Autodesk Inventor part; units mm, degrees
ref_plane "YZ Plane" through (0, 0, 0) normal (1, 0, 0) x (0, 1, 0)
ref_plane "XZ Plane" through (0, 0, 0) normal (0, 1, 0) x (-1, 0, 0)
ref_plane "XY Plane" through (0, 0, 0) normal (0, 0, 1) x (1, 0, 0)
sketch "Sketch1" plane through (0, 0, 0) normal (0, 1, 0) x (-1, 0, 0)
  line L0 (-23.8125, -82.566) -> (23.8125, -82.566)
  line L1 (23.8125, -82.566) -> (23.8125, 82.566)
  line L2 (23.8125, 82.566) -> (-23.8125, 82.566)
  line L3 (-23.8125, 82.566) -> (-23.8125, -82.566)
  line L4 (-23.8125, -82.566) -> (23.8125, 82.566) construction
  line L5 (23.8125, -82.566) -> (-23.8125, 82.566) construction
  point P0 (0, 0)
  dimension "d0" = 47.625
  dimension "d1" = 165.132
extrude "Extrusion1" add sketch "Sketch1" along normal blind 20.6248
sketch "Sketch5" plane through (-23.8125, 0, -82.566) normal (-1, 0, 0) x (0, 0, 1)
  line L0 (0, 20.6248) -> (165.132, 20.6248)
  line L1 (165.132, 0) -> (0, 0)
  line L2 (0, 20.6248) -> (165.132, 20.6248)
  line L3 (165.132, 20.6248) -> (165.132, 0)
  line L4 (165.132, 0) -> (0, 0)
  line L5 (0, 0) -> (0, 20.6248)
  point P0 (82.566, 0)
extrude "Extrusion4" add sketch "Sketch5" along normal blind 2.3495
sketch "Sketch6" plane through (23.8125, 0, 82.566) normal (1, 0, 0) x (0, 0, -1)
  line L0 (0, 0) -> (0, 20.6248)
  line L1 (0, 0) -> (165.132, 0)
  line L2 (0, 20.6248) -> (165.132, 20.6248)
  line L3 (165.132, 20.6248) -> (165.132, 0)
  line L4 (165.132, 0) -> (0, 0)
  line L5 (0, 0) -> (0, 20.6248)
  point P0 (82.566, 0)
extrude "Extrusion5" add sketch "Sketch6" along normal blind 2.3495
sketch "Sketch7" plane through (-26.162, 0, -82.566) normal (0, 0, -1) x (-1, 0, 0)
  line L0 (0, 0) -> (-52.324, 0)
  line L1 (0, -3.175) -> (3.175, -3.175)
  line L2 (0, -3.175) -> (0, 0)
  arc A0 (3.175, -3.175) -> (0, 0) centre (0, -3.175) ccw
  line L3 (-52.324, 0) -> (-52.324, -3.175)
  arc A1 (-52.324, 0) -> (-55.499, -3.175) centre (-52.324, -3.175) ccw
  line L4 (-52.324, -3.175) -> (-55.499, -3.175)
  line L5 (-52.324, 0) -> (-52.324, 6.35)
  line L6 (-52.324, 0) -> (-52.324, 20.6248)
  arc A2 (-52.324, 6.35) -> (-61.849, -3.175) centre (-52.324, -3.175) ccw
  line L7 (-55.499, -3.175) -> (-61.849, -3.175)
  line L8 (-55.499, -3.175) -> (-55.499, -10.795)
  line L9 (-55.499, -10.795) -> (-61.849, -10.795)
  line L10 (-61.849, -10.795) -> (-61.849, -3.175)
  line L11 (-55.499, -10.795) -> (-58.674, -10.795)
  arc A3 (-58.674, -13.97) -> (-55.499, -10.795) centre (-58.674, -10.795) ccw
  line L12 (-58.674, -13.97) -> (-66.294, -13.97)
  line L13 (-66.294, -13.97) -> (-66.294, -17.145)
  arc A4 (-66.294, -13.97) -> (-69.469, -17.145) centre (-66.294, -17.145) ccw
  line L14 (-66.294, -17.145) -> (-69.469, -17.145)
  line L15 (-69.469, -17.145) -> (-69.469, -22.225)
  line L16 (-61.849, -13.97) -> (-61.849, -7.62)
  line L17 (-61.849, -7.62) -> (-66.294, -7.62)
  arc A5 (-66.294, -7.62) -> (-75.819, -17.145) centre (-66.294, -17.145) ccw
  line L18 (-69.469, -22.225) -> (-75.819, -22.225)
  line L19 (-75.819, -22.225) -> (-75.819, -17.145)
  line L20 (-69.469, -17.145) -> (-75.819, -17.145)
  line L21 (-26.162, 0) -> (-26.162, 12.6356)
  arc A6 (3.175, -3.175) -> (0, 0) centre (0, -3.175) ccw
  line L22 (0, -3.175) -> (3.175, -3.175)
  arc A7 (9.525, -3.175) -> (0, 6.35) centre (0, -3.175) ccw
  line L23 (3.175, -3.175) -> (9.525, -3.175)
  line L24 (3.175, -3.175) -> (3.175, -10.795)
  line L25 (3.175, -10.795) -> (9.525, -10.795)
  line L26 (9.525, -10.795) -> (9.525, -3.175)
  line L27 (3.175, -10.795) -> (6.35, -10.795)
  arc A8 (3.175, -10.795) -> (6.35, -13.97) centre (6.35, -10.795) ccw
  line L28 (6.35, -13.97) -> (13.97, -13.97)
  line L29 (13.97, -13.97) -> (13.97, -17.145)
  arc A9 (17.145, -17.145) -> (13.97, -13.97) centre (13.97, -17.145) ccw
  line L30 (13.97, -17.145) -> (17.145, -17.145)
  line L31 (17.145, -17.145) -> (17.145, -22.225)
  line L32 (9.525, -13.97) -> (9.525, -7.62)
  line L33 (9.525, -7.62) -> (13.97, -7.62)
  arc A10 (23.495, -17.145) -> (13.97, -7.62) centre (13.97, -17.145) ccw
  line L34 (17.145, -22.225) -> (23.495, -22.225)
  line L35 (23.495, -22.225) -> (23.495, -17.145)
  line L36 (17.145, -17.145) -> (23.495, -17.145)
  line L37 (0, 20.6248) -> (0, 0)
  line L38 (0, 0) -> (0, 6.35)
  dimension "d22" = 3.175
  dimension "d23" = 6.35
  dimension "d24" = 7.62
  dimension "d26" = 7.62
  dimension "d29" = 3.175
  dimension "d30" = 5.08
  dimension "d31" = 6.35
  dimension "d32" = 6.35
extrude "Extrusion6" add sketch "Sketch7" against normal blind 158.75 contours A1 L7 A2 L5 | L37 A7 L23 A0 | L23 L26 L25 L24 | L25 L32 L28 A8 | L8 L9 L10 L7 | L33 A10 L36 A9 L28 L32 L26 | A3 L12 L16 L9 | L10 L16 L12 A4 L20 A5 L17 | L35 L34 L31 L36 | L20 L15 L18 L19
sketch "Sketch10" plane through (-26.162, 0, 82.566) normal (0, 0, 1) x (1, 0, 0)
  line L0 (26.162, 20.0804) -> (26.162, 7.3804)
  line L1 (26.162, 7.3804) -> (38.862, 7.3804)
  line L2 (26.162, 7.3804) -> (13.462, 7.3804)
  circle A0 centre (13.462, 7.3804) radius 3.5687
  circle A1 centre (38.862, 7.3804) radius 3.5687
  point P0 (26.162, 0)
  dimension "d52" = 12.7
  dimension "d53" = 12.7
  dimension "d54" = 12.7
  dimension "d55" = 7.1374
  dimension "d56" = 7.1374
extrude "Extrusion9" cut sketch "Sketch10" against normal blind 6.35
sketch "Sketch11" plane through (26.162, 20.6248, -82.566) normal (0, 0, -1) x (-1, 0, 0)
  line L0 (0, 0) -> (52.324, 0)
  line L1 (26.162, 0) -> (26.162, -12.7)
  line L2 (26.162, -12.7) -> (38.862, -12.7)
  line L3 (38.862, -12.7) -> (13.462, -12.7)
  circle A0 centre (38.862, -12.7) radius 3.5687
  circle A1 centre (13.462, -12.7) radius 3.5687
  point P0 (26.162, -20.6248)
  dimension "d59" = 12.7
  dimension "d60" = 12.7
  dimension "d61" = 25.4
  dimension "d62" = 7.1374
  dimension "d63" = 7.1374
extrude "Extrusion10" cut sketch "Sketch11" against normal blind 6.35
properties part number "Clamp connector"
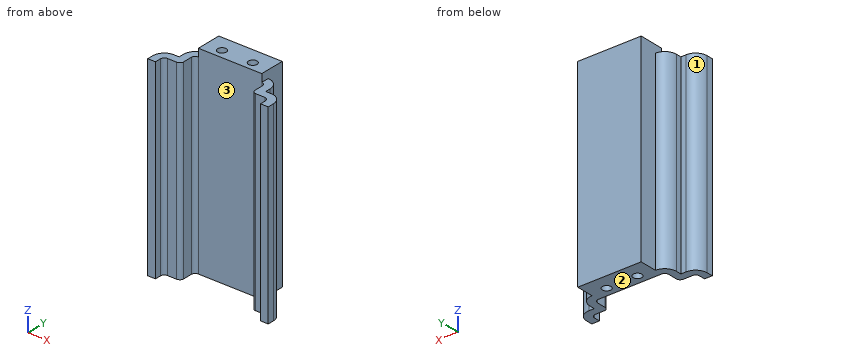
Geometry: final body of the model. Coordinates: model frame, mm. Face numbers are marked on the shaded views. Give positions to 0.01 mm unless a question says otherwise; leave off trailing zeros. Loops run counter-clockwise (first coordinate to the right, second up) from the corner with the lowest first, then second, coordinate; pieces in that order, holes last. Notation, with made-up numbers: (66, 60) -> (108, 60) arc R22 ccw to (108, 85) -> close; hole circle Ø3 at (-5.5, -29). An arc over 180 degrees is marked (long way). Put each result on its own line as item: value.
1. Cut plane A-A (x = -12.7). Return the cut outline in (y, z).
Taken from the geometry:
outline: (0, -82.57) -> (4.36, -82.57) -> (4.36, -76.22) -> (11.49, -76.22) -> (11.49, -82.57) -> (20.62, -82.57) -> (20.62, 82.57) -> (10.95, 82.57) -> (10.95, 76.22) -> (3.81, 76.22) -> (3.81, 82.57) -> (0, 82.57) -> close
2. Pull-direction query (X, two-part tool) for the marked faces 1, 2 and 3; classes: released by +X, released by -X, zero draft, split by the parting line, or undercut.
Taken from the geometry:
face 1: released by -X
face 2: zero draft
face 3: undercut
3. Ray query, line 1 along Y through (x, z) = (-12.7, -77.75); line 2 along Y through (x, z) = (-12, -80); line 3 along Y through (x, z) = (16.5, -6.5). Return the intervals inside material, ascending. Write a range as [from, to].
Taken from the geometry:
line 1: y = [0, 4.36], [11.49, 20.62]
line 2: y = [0, 4.43], [11.42, 20.62]
line 3: y = [0, 20.62]
4. Cut plane B-B (z = -27). Return the cut outline in (x, y) (3 decimals).
Taken from the geometry:
outline: (-49.657, -22.225) -> (-43.307, -22.225) -> (-43.307, -17.145) arc R3.175 cw to (-40.132, -13.97) -> (-32.512, -13.97) arc R3.175 ccw to (-29.337, -10.795) -> (-29.337, -3.175) arc R3.175 cw to (-26.162, 0) -> (26.162, 0) arc R3.175 cw to (29.337, -3.175) -> (29.337, -10.795) arc R3.175 ccw to (32.512, -13.97) -> (40.132, -13.97) arc R3.175 cw to (43.307, -17.145) -> (43.307, -22.225) -> (49.657, -22.225) -> (49.657, -17.145) arc R9.525 ccw to (40.132, -7.62) -> (35.687, -7.62) -> (35.687, -3.175) arc R9.525 ccw to (26.162, 6.35) -> (26.162, 20.625) -> (-26.162, 20.625) -> (-26.162, 6.35) arc R9.525 ccw to (-35.687, -3.175) -> (-35.687, -7.62) -> (-40.132, -7.62) arc R9.525 ccw to (-49.657, -17.145) -> close
5. Cut plane C-C (y = 17). Return the cut outline in (x, z).
Taken from the geometry:
outline: (-26.16, -82.57) -> (26.16, -82.57) -> (26.16, 82.57) -> (-26.16, 82.57) -> close
6. Pin query (flat end, axial travel): P1, Ø1.5, axis at x = 9.5, z = -56.5, coming from the -Y side; P2, Ø10, axis at y = -14, z = 44.5, coming from the -X side; P3, Ø4, axis at x = 34.5, z = 7, coming from the -Y side; P4, Ø6.5, axis at x = 12.7, y = 7.92, coming from the -Z side. Return the tip coordinate at first contact, or that it passes through.
Taken from the geometry:
P1: stops at y = 0
P2: stops at x = -49.66
P3: stops at y = -13.97
P4: stops at z = -76.22
7. Cut plane D-D (x = 5). Return the cut outline in (y, z).
Taken from the geometry:
outline: (0, -82.57) -> (20.62, -82.57) -> (20.62, 82.57) -> (0, 82.57) -> close
